Geometry check sheet. Reference: drawing and pictorial views, mm from the part's lowest x, y, z. A direction names the side the tool comes from. Coordinates: 2 decimals unless noted, no trailing zeros. Write each loop counter-clockwise with the first axis right and the second up, starting at its lowest first coordinate (ties: lowest second). Pieces come first, ordered by that corner, then holes. Notation, with made-up numbers: (11.25, 55) -> (25.25, 55) arc R26 ccw to (25.25, 81) -> close; hole circle Ø10 at (20.5, -34). An arc over 180 degrees is marked (long way). Use a Markdown table: item, result.
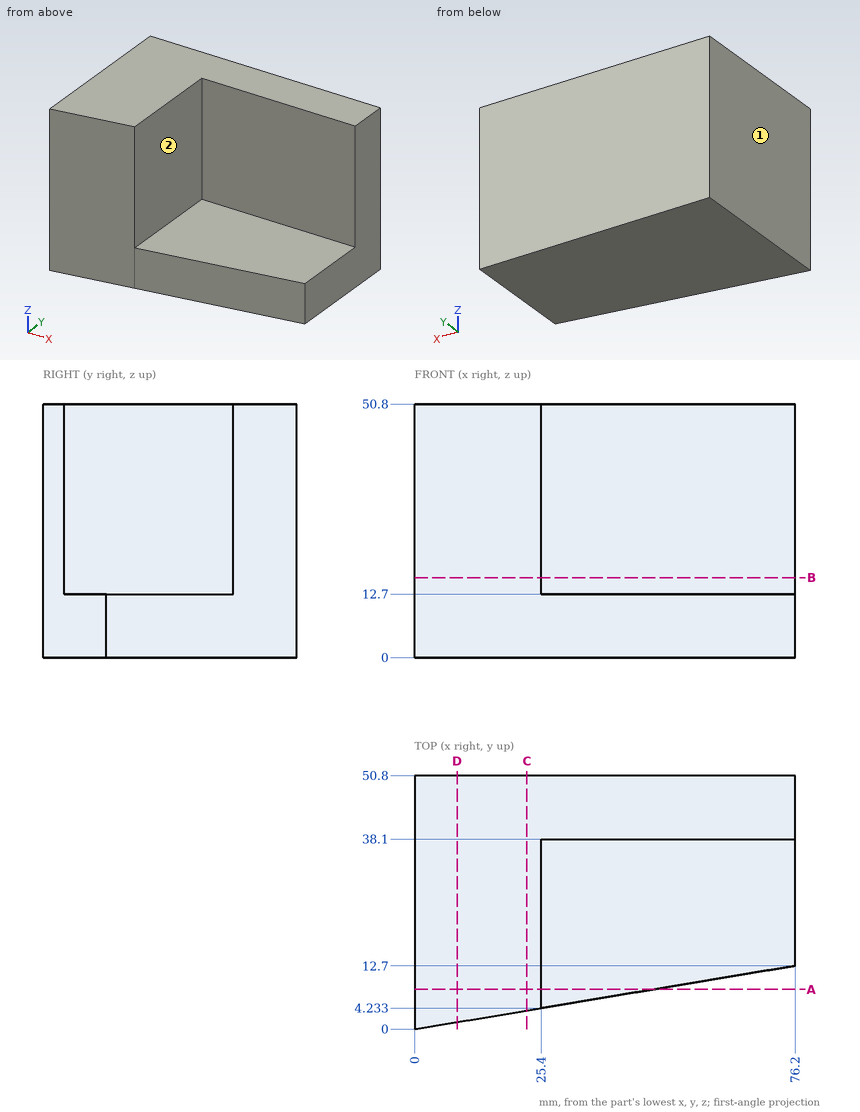
Item 1: Section check D-D on x = 8.5. Record the boundary of the cut face in (y, z), then the cut area to 3 significant figures.
Answer block:
| item | result |
|---|---|
| outline | (1.42, 0) -> (50.8, 0) -> (50.8, 50.8) -> (1.42, 50.8) -> close |
| area | 2,510 mm^2 |
Item 2: Section check C-C on x = 22.5. Record the boundary of the cut face in (y, z), then the cut area to 3 significant figures.
Answer block:
| item | result |
|---|---|
| outline | (3.75, 0) -> (50.8, 0) -> (50.8, 50.8) -> (3.75, 50.8) -> close |
| area | 2,390 mm^2 |
Item 3: Thickness scan on L1, parallel to X at y = 6, z = 47.5; L2, parallel to Y at x = 46.5, z = 40.5; L3, parallel to Z at x = 72, y = 24. Record the ranges inside material, lowest first. Write a range as [from, to].
Answer block:
| item | result |
|---|---|
| L1 | x = [0, 25.4] |
| L2 | y = [38.1, 50.8] |
| L3 | z = [0, 12.7] |
Item 4: Section check A-A on y = 8. Record the boundary of the cut face in (x, z).
Answer block:
| item | result |
|---|---|
| outline | (0, 0) -> (48, 0) -> (48, 12.7) -> (25.4, 12.7) -> (25.4, 50.8) -> (0, 50.8) -> close |
Item 5: Depth check by flat-ended pin: P1, Ø1.5, axis at x = 41.5, y = 24, coming from the -Z side; P2, Ø3, axis at y = 9.5, z = 31, coming from the +X side; P3, Ø6, axis at x = 25, z = 20, coming from the -Y side. Enter the tip coordinate at first touch or a pass-through.
Answer block:
| item | result |
|---|---|
| P1 | stops at z = 0 |
| P2 | stops at x = 25.4 |
| P3 | stops at y = 3.67 |
Item 6: Tool access check on the marked faces 1 and 2. Record the directions out of +Z, -Z, +X, -X, +Y, -Y that give a thin tool (end or side, any length) a straight path to the whole face; none if there is none.
Answer block:
| item | result |
|---|---|
| face 1 | +Z, -Z, -X, +Y, -Y |
| face 2 | +Z, +X, -Y |
Item 7: Section check B-B on z = 16. Record the boundary of the cut face in (x, y), then the cut area to 3 significant figures.
Answer block:
| item | result |
|---|---|
| outline | (0, 0) -> (25.4, 4.23) -> (25.4, 38.1) -> (76.2, 38.1) -> (76.2, 50.8) -> (0, 50.8) -> close |
| area | 1,880 mm^2 |
